Can you work these out from the model? Positions are in its coordinate system, mm. A direction names the side the tool comes from. Give positions to 0.01 mm unless a question says otherwise; leave off trailing zeros. Loops run counter-clockwise (first coordinate to the right, second up) from the corner with the lowest first, then second, coordinate; pieces in that order, holes last. Notation, with made-up numbers: (42.5, 14) - (82.5, 14) arc R6 ccw to (82.5, 25) - close; hole circle Ø9 at (81, -31). An arc over 180 degrees is marked (long way). Answer as a JSON object with one key per item and string values. Group by question number.
Item 1: Suppose I cut it at A-A on x = 0. Write out the boundary of the cut face in (y, z), and give its area (3 significant figures).
Item 2: Which directions (+Z, -Z, +X, -X, +Y, -Y) give clear straight access to the entire face, cutting with the end or side of a thin tool? Please do faces 4 (the flat face through (2, 0.6, 7)), 5 (the flat face through (-3.92, 0, 1.42)).
Item 3: Thinking about a two-plate mould opening in X: for faces 1 (the cylindrical face through (3.563, 1.978, 0.468)), 2 (the flat face through (-4, 4, -2)), 3 (the cylindrical face through (9.76, 2.32, 2.17)), which applies, pulls with the +X half, pulls with the -X half, needs draft (parallel to the pull), parting line crosses it, or undercut?
Item 4: Suppose I cut it at B-B on z = 0. Write out the boundary of the cut face in (x, y), and give its area (3 significant figures).
Item 5: Will these pins go through, and if not, where does the flat tip stop? pin 1 (1 mm diameter, centred on x = 6.5, y = 2.5, fed in from -Z); pin 2 (1 mm diameter, centred on y = 3.5, z = 1.5, fed in from +X).
Item 6: Please list where these lines run through material, in increasing order: L1, parallel to X at y = 2.85, z = 0; L2, parallel to Y at x = -6.75, z = 3; L3, parallel to X at y = 2.5, z = -2.5.
Autodesk Inventor part; units mm, degrees
ref_plane "ANBAU_XY" through (0, 0, 0) normal (0, 1, 0) x (1, 0, 0)
ref_plane "ANBAU_YZ" through (0, 0, 0) normal (1, 0, 0) x (0, 0, -1)
ref_plane "ANBAU_ZX" through (0, 0, 0) normal (0, 0, -1) x (0, 1, 0)
sketch "Sketch_1" plane through (0, 0, 0) normal (1, 0, 0) x (0, 1, 0)
  line L0 (0, 0) -> (4, 0)
  line L1 (0.406, -3.594) -> (0, -4)
  line L2 (0, -4) -> (0, -6)
  arc A0 (0.6, -6.9165) -> (0, -6) centre (-0.4, -6.9165) ccw
  line L3 (0.6, -6.9165) -> (0.6, -9.6)
  line L4 (0.6, -9.6) -> (1, -10)
  line L5 (1, -10) -> (3.6, -10)
  line L6 (3.6, -10) -> (4, -9.6)
  line L7 (4, -9.6) -> (4, -4)
  line L8 (4, -4) -> (3.594, -3.594)
  line L9 (3.594, -3.594) -> (0.406, -3.594)
revolve "Revolution1" add sketch "Sketch_1" angle 360 about axis through (0, 0, 0) along (0, -1, 0)
thread "Thread1"
ref_plane "ANBAU_XY" through (0, 0, 0) normal (0, 1, 0) x (1, 0, 0)
ref_plane "ANBAU_YZ" through (0, 0, 0) normal (1, 0, 0) x (0, 0, -1)
ref_plane "ANBAU_ZX" through (0, 0, 0) normal (0, 0, -1) x (0, 1, 0)
properties part number "209407 M8X0,75"
Worked out:
{
 "1": {"outline": "(0, -6) arc R1 cw to (0.6, -6.92) - (0.6, -9.6) - (1, -10) - (3.6, -10) - (4, -9.6) - (4, -4) - (3.59, -3.59) - (0.41, -3.59) - (0, -4) - close; (0, 4) - (0.41, 3.59) - (3.59, 3.59) - (4, 4) - (4, 9.6) - (3.6, 10) - (1, 10) - (0.6, 9.6) - (0.6, 6.92) arc R1 cw to (0, 6) - close", "area": "46.1 mm2"},
 "2": {"face 4": "-Y", "face 5": "+Z, -Z, +X, -X, -Y"},
 "3": {"face 1": "undercut", "face 2": "needs draft", "face 3": "parting line crosses it"},
 "4": {"outline": "(-10, 1) - (-9.6, 0.6) - (-6.92, 0.6) arc R1 cw to (-6, 0) - (-4, 0) - (-3.59, 0.41) - (-3.59, 3.59) - (-4, 4) - (-9.6, 4) - (-10, 3.6) - close; (3.59, 0.41) - (4, 0) - (6, 0) arc R1 cw to (6.92, 0.6) - (9.6, 0.6) - (10, 1) - (10, 3.6) - (9.6, 4) - (4, 4) - (3.59, 3.59) - close", "area": "46.1 mm2"},
 "5": {"pin 1": "stops at z = -8", "pin 2": "stops at x = 9.95"},
 "6": {"L1": "x = -10 to -3.59, 3.59 to 10", "L2": "y = 0.6 to 4", "L3": "x = -9.68 to -2.58, 2.58 to 9.68"}
}
